Design review of the part built by this model. Coordinates are the model's own, in mm. A direction names the side the tool comes from. Round coordinates to 2 decimals unless told otherwise and drop trailing zeros. Loops run counter-clockwise (first coordinate to the right, second up) from the corner with the lowest first, then second, coordinate; pieces in that order, holes last. Notation, with made-up numbers: (-18.75, 58) -> (26.25, 58) arc R12 cw to (26.25, 76) -> close; hole circle Ø3 at (3, 29). An arc over 180 degrees is marked (long way). Use a Markdown table: item, result. Add a question column.
from build123d import *


with BuildPart() as part:
    # Sketch1 → Revolve1 (revolve)
    with BuildSketch(Plane(origin=(0, 0, 0), x_dir=(0, 0, -1), z_dir=(1, 0, 0)), mode=Mode.PRIVATE) as revolve1_sk:
        with BuildLine():
            Line((-0.127, 6.35), (-0.127, 7.9375))
            Line((-0.127, 7.9375), (-9.525, 7.9375))
            Line((-9.525, 7.9375), (-9.525, 10.649273743))
            ThreePointArc((-9.525, 10.649273743), (-10.834561548, 9.313695954), (-11.958424774, 7.818486629))
            ThreePointArc((-11.958424774, 7.818486629), (-12.487029733, 7.470791715), (-13.10188894, 7.62))
            Line((-13.10188894, 7.62), (-19.812, 12.7))
            Line((-19.812, 12.7), (-22.987, 12.7))
            Line((-22.987, 12.7), (-22.987, 6.35))
            Line((-22.987, 6.35), (-0.127, 6.35))
        make_face()
    revolve(revolve1_sk.sketch.rotate(Axis((0, 0, 47.275745838), (0, 0, -1)), 90), axis=Axis((0, 0, 47.275745838), (0, 0, -1)))


solid = part.part
1. Consider section C-C on z = 21. State the section outline as (x, y) points, plus the area to 3 significant figures.
2. To check wall thickness, follow probe 1 along Y at (x, z) = (0, 9.25); probe 2 along Z at (x, y) = (5, -7.5) (3 decimals); probe 3 along Y at (x, z) = (0, 18). State the ranges of each line that lie inside material, in increasing order. Write a range as from..to.
3. Mouldability with a two-part tool opening along Y and no side actions: class faces 4 (the face through (2, -8, 9.525)), 5 (the face through (-5.04, 3.86, 11.4)), 6 (the face through (-10.1, 7.7, 21.4)) as +Y half, -Y half, draft (parallel to the pull), parting line (faces both ways), or undercut.
4. For faces 1 (the face through (-1.72, 7.75, 4.89)), 2 (the face through (3.66, 7.04, 13.52)), 3 (the face through (3, -6, 22.987)), list the 3-axis set-ups (+Z, -Z, +X, -X, +Y, -Y) from which the entire face can be reached by the end or side of a thin tool; tool diameter is ignored.
5. Insertion check: P1, Ø3, axis at x = 2, z = 15, coming from the -Y side; P2, Ø1, axis at x = -5.5, y = 9, coming from the -Z side (3 decimals); P3, Ø6, axis at x = 5, z = 4.5, coming from the -Y side. Each pin has a flat end and moves straight along its axis. Give the tip position at first contact, or say it passes through.
Verdict:
| question | item | result |
|---|---|---|
| 1 | outline | circle Ø25.4 at (0, 0); hole circle Ø12.7 at (0, 0) |
| 1 | area | 380 mm² |
| 2 | probe 1 | y = -7.94..-6.35, 6.35..7.94 |
| 2 | probe 2 | z = 9.525..11.085, 14.943..22.987 |
| 2 | probe 3 | y = -11.33..-6.35, 6.35..11.33 |
| 3 | face 4 | draft |
| 3 | face 5 | undercut |
| 3 | face 6 | parting line |
| 4 | face 1 | -Z |
| 4 | face 2 | none |
| 4 | face 3 | +Z, +X, -X, +Y, -Y |
| 5 | P1 | stops at y = -10.03 |
| 5 | P2 | stops at z = 9.525 |
| 5 | P3 | stops at y = -7.68 |
